```python
from build123d import *

# Parameters (mm, degrees)
BOSS_EXTRU_1_DEPTH      = 60
ENL_V_START             = 1.589213588
ENL_V_MAT_EXTRU_1_DEPTH = 60.853997617
CONG_1_R                = 5


# Read off the part's stored shape, not the designer's step: Enlèv. mat.-Extru.1
with BuildPart() as part:
    # Esquisse1 → Boss.-Extru.1 (new body)
    with BuildSketch(Plane.XY):
        Polygon((0, 0), (60, 0), (60, 23.8), (35, 23.8), (35, 30.8), (60, 45.8), (60, 60), (0, 60), (0, 45.8), (25, 30.8), (25, 23.8), (0, 23.8), align=None)
    extrude(amount=BOSS_EXTRU_1_DEPTH)

    # Enlèv. mat.-Extru.1 outline → Enlèv. mat.-Extru.1 (cut)
    with BuildSketch(Plane(origin=(0, 0, 0), x_dir=(1, 0, 0), z_dir=(0, 0.05159784377706792, 0.9986679440722813)).offset(ENL_V_START)):
        Polygon((60, 45.738991839), (35, 30.758972677), (35, 26), (60, 26), align=None)
        Polygon((0, 26), (25, 26), (25, 30.758972677), (0, 45.738991839), align=None)
    extrude(amount=ENL_V_MAT_EXTRU_1_DEPTH, mode=Mode.SUBTRACT)

    # Congé1
    cong_1_edges = [part.edges().sort_by_distance(p)[0] for p in [
        (30, 0, 0),
        (30, 0, 60),
    ]]
    fillet(cong_1_edges, radius=CONG_1_R)


solid = part.part
```
Input: part model. Units: mm. Frame: model coordinates. A direction names the side the tool comes from. Round coordinates to 2 decimals unless told otherwise and drop trailing zeros. Order: outer loops, then holes, each group sorted by start corner. A loop starts at its lowest first (then second) coordinate and runs counter-clockwise, first axis right, second up. Notation, with made-up numbers: (41, 9.5) - (68, 9.5) arc R9 ccw to (68, 18.5) - close; hole circle Ø4 at (-33.75, 5.5). An arc over 180 degrees is marked (long way). One line per question, with ' | ' between items. Start each with the question number.
1) Pull-direction query (Y, two-part tool) for faces 1 (the flat face through (30, 60, 30)), 2 (the flat face through (13, 23.8, 30)), 3 (the flat face through (30, 33, 0)); classes: +Y half, -Y half, draft (parallel to the pull), parting line (faces both ways), or undercut.
2) Cut plane C-C, the plane z = 12. Return the cut outline in (x, y).
3) Contact query for flat-ended pins moving along their axis: P1, Ø5, axis at y = 26.5, z = 28.5, coming from the -X side; P2, Ø2, axis at y = 16, z = 8.5, coming from the -X side; P3, Ø6, axis at x = 43.5, y = 28.5, coming from the +Z side; P4, Ø5, axis at y = 30, z = 44, coming from the +X side. Output: stop coordinate, or through.
4) Cut plane A-A, the plane x = 45. Return the cut outline in (y, z), then the cut area to 3 significant figures.
5) Cut plane B-B, the plane x = 51.5. Return the cut outline in (y, z), then the cut area to 3 significant figures.
6) Cut plane D-D, the plane y = 25. Return the cut outline in (x, z), then the cut area to 3 significant figures.
7) Ray query, probe 1 along X at (y, z) = (30, 12); probe 2 along Y at (x, z) = (12, 10.5); probe 3 along Y at (x, z) = (42, 51) (3 decimals). Return the intervals inside material, ascending.
8) Set-up query: faces 4 (the flat face through (47.675, 39.933, 29.569)), 5 (the flat face through (12.675, 39.723, 29.58)), 6 (the flat face through (48, 23.8, 30)). Return all of +Z, -Z, +X, -X, +Y, -Y with unobstructed straight access to the full face (end or side cutting, diameter ignored); none if empty.
Worked out:
1) face 1: +Y half | face 2: undercut | face 3: draft
2) outline: (0, 0) - (60, 0) - (60, 23.8) - (35, 23.8) - (35, 31.42) - (60, 46.42) - (60, 60) - (0, 60) - (0, 46.42) - (25, 31.42) - (25, 23.8) - (0, 23.8) - close
3) P1: stops at x = 25 | P2: stops at x = 0 | P3: passes through | P4: stops at x = 35
4) outline: (0, 5) arc R5 ccw to (5, 0) - (23.8, 0) - (23.8, 60) - (5, 60) arc R5 ccw to (0, 55) - close; (36.8, 0) - (60, 0) - (60, 60) - (39.9, 60) - close | area: 2,720 mm^2
5) outline: (0, 5) arc R5 ccw to (5, 0) - (23.8, 0) - (23.8, 60) - (5, 60) arc R5 ccw to (0, 55) - close; (40.7, 0) - (60, 0) - (60, 60) - (43.8, 60) - close | area: 2,480 mm^2
6) outline: (25, 0) - (35, 0) - (35, 60) - (25, 60) - close | area: 600 mm^2
7) probe 1: x = 25 to 35 | probe 2: y = 0 to 23.8, 39.14 to 60 | probe 3: y = 0 to 23.8, 37.635 to 60
8) face 4: +Z, +X | face 5: +Z, -X | face 6: +Z, -Z, +X
